```python
from build123d import *
from OCP.BRepFilletAPI import BRepFilletAPI_MakeChamfer

# Parameters (mm, degrees)
F_41_64_0_640630_DIAMETER_HOLE1_D = 16.272002
SKETCH7_W                         = 76.989658396
SKETCH7_H                         = 50.8
FCE_00_BOLT_HEAD_NOTCH_DEPTH      = 50.8
FILLET1_R                         = 3.175
CHAMFER1_SIZE                     = 0.381
CHAMFER1_SIZE2                    = 0.387827593
CUT_EXTRUDE1_DEPTH                = 110.652296603
CUT_EXTRUDE1_DEPTH_BACK           = 110.652296603


with BuildPart() as part:
    # Sketch3 → FBR-00 Basic blank revolve. (revolve)
    with BuildSketch(Plane(origin=(0, 0, 0), x_dir=(0, 0, -1), z_dir=(1, 0, 0)), mode=Mode.PRIVATE) as fbr_00_basic_blank_revolve_sk:
        with BuildLine():
            Line((-101.188905116, 30.1625), (-101.188905116, 0))
            Line((-101.188905116, 0), (-21.038993491, 0))
            Line((-21.038993491, 0), (-6.731, 23.8125))
            Line((-6.731, 23.8125), (9.144, 23.8125))
            Line((9.144, 23.8125), (9.144, 28.448))
            Line((9.144, 28.448), (6.096, 28.448))
            Line((6.096, 28.448), (4.602815367, 26.954815367))
            ThreePointArc((4.602815367, 26.954815367), (4.064, 26.731630735), (3.525184633, 26.954815367))
            Line((3.525184633, 26.954815367), (2.032, 28.448))
            Line((2.032, 28.448), (0, 28.448))
            Line((0, 28.448), (0, 29.21))
            Line((0, 29.21), (-2.286, 29.21))
            Line((-2.286, 29.21), (-3.2385, 30.1625))
            Line((-3.2385, 30.1625), (-101.188905116, 30.1625))
        make_face()
    revolve(fbr_00_basic_blank_revolve_sk.sketch.rotate(Axis((0, 0, -27.766671499), (0, 0, 1)), 90), axis=Axis((0, 0, -27.766671499), (0, 0, 1)))

    # Sketch13 → FCR-00 lacation boss, Cut-Revolve. (revolve, cut)
    with BuildSketch(Plane(origin=(0, 0, 0), x_dir=(0, 0, -1), z_dir=(1, 0, 0))):
        Polygon((-60.009409083, 44.720607894), (-79.306268956, 26.150824711), (-82.534005377, 29.389847768), (-90.632639597, 21.596357919), (-105.074812876, 36.603996473), (-77.621815521, 63.022606131), align=None)
    revolve(axis=Axis((0, 36.603996473, 105.074812876), (0, 0.720551111680328, 0.6934018282758155)), mode=Mode.SUBTRACT)

    # 41/64 (0.640630) Diameter Hole1 (through all)
    with Locations(Plane(origin=(0, 56.495615275, 54.366945365), x_dir=(1, 0, 0), z_dir=(0, 0.720551111680328, 0.6934018282758155))):
        with Locations((0, -50.330495151)):
            Hole(F_41_64_0_640630_DIAMETER_HOLE1_D / 2)

    # FCS-00 End trim, Cut-Sweep: sweep along a path in Sketch6
    with BuildLine(Plane(origin=(0, 53.201255592, 51.196712206), x_dir=(1, 0, 0), z_dir=(0, 0.720551111680328, 0.6934018282758155))) as fcs_00_end_trim_cut_sweep_path:
        Line((-25.4, -39.765602031), (-25.4, -52.465602031))
        ThreePointArc((-25.4, -52.465602031), (-23.103230962, -59.750022773), (-17.04365582, -64.399698315))
        Line((-17.04365582, -64.399698315), (-6.51548373, -68.231639577))
        ThreePointArc((-6.51548373, -68.231639577), (-3.307997785, -69.091082846), (0, -69.380495151))
    # Sketch16 → FCS-00 End trim, Cut-Sweep (sweep, cut)
    with BuildSketch(Plane(origin=(0, 117.771567215, -110.982310617), x_dir=(0, -0.9982398279237649, -0.059306373575968775), z_dir=(-1, 0, 0))):
        with BuildLine():
            Line((152.30720814, 182.06896008), (168.803188567, 201.383271607))
            Line((168.803188567, 201.383271607), (110.860253989, 250.871212889))
            Line((110.860253989, 250.871212889), (88.178280901, 224.314034541))
            Line((88.178280901, 224.314034541), (97.835436664, 216.066044327))
            Line((97.835436664, 216.066044327), (99.302186796, 217.783388083))
            ThreePointArc((99.302186796, 217.783388083), (99.979412877, 218.248832673), (100.798630163, 218.313306472))
            Line((100.798630163, 218.313306472), (112.384771543, 216.165942094))
            Line((112.384771543, 216.165942094), (152.30720814, 182.06896008))
        make_face()
    fcs_00_end_trim_cut_sweep = sweep(path=fcs_00_end_trim_cut_sweep_path.line, mode=Mode.SUBTRACT)

    # FMR-00 Mirror end trim.: FCS-00 End trim, Cut-Sweep across plane
    add(fcs_00_end_trim_cut_sweep.mirror(Plane(origin=(0, 0, 0), x_dir=(0, 0, 1), z_dir=(1, 0, 0))), mode=Mode.SUBTRACT)

    # Sketch7 → FCE-00 Bolt head notch. (cut)
    with BuildSketch(Plane(origin=(0, -18.301998237, 52.237593562), x_dir=(1, 0, 0), z_dir=(0, -0.7205511116803286, -0.6934018282758149))):
        with Locations((0, 6.35)):
            Rectangle(SKETCH7_W, SKETCH7_H)
    extrude(amount=FCE_00_BOLT_HEAD_NOTCH_DEPTH, mode=Mode.SUBTRACT)

    # Fillet1
    fillet1_edges = [part.edges().sort_by_distance(p)[0] for p in [
        (0, -5.092693408, 38.511094884),
    ]]
    fillet(fillet1_edges, radius=FILLET1_R)

    # Chamfer1: one chamfer whose edges measure the first distance from different faces: ONE call of the kernel's chamfer builder (chamfer() names one face for all edges)
    chamfer1_edges_1 = [part.edges().sort_by_distance(p)[0] for p in [
        (28.448, 0, -9.144),
        (23.8125, 0, -9.144),
    ]]
    chamfer1_edges_2 = [part.edges().sort_by_distance(p)[0] for p in [
        (0, 13.80286807, 98.731273817),
    ]]
    chamfer1_side_2 = [part.faces().sort_by_distance(p)[0] for p in [
        (0, 14.023301251, 98.50220985),
    ]]
    chamfer1 = BRepFilletAPI_MakeChamfer(part.part.solid().wrapped)
    for e in chamfer1_edges_1:
        chamfer1.Add(CHAMFER1_SIZE, e.wrapped)
    for e in chamfer1_edges_2:
        chamfer1.Add(CHAMFER1_SIZE, CHAMFER1_SIZE2, e.wrapped, chamfer1_side_2[0].wrapped)  # the first distance lies on this face
    add(Compound.cast(chamfer1.Shape()), mode=Mode.REPLACE)

    # Sketch17 → Cut-Extrude1 (cut, two sides: drawn at the far end of the back side and taken through both)
    with BuildSketch(Plane(origin=(0, 0, 0), x_dir=(0, 0, -1), z_dir=(1, 0, 0)).offset(-CUT_EXTRUDE1_DEPTH_BACK)):
        Polygon((-220.872013196, 249.233244147), (-107.294691274, 15.329981457), (-88.096461038, -24.20721324), (25.480860884, -258.110475929), (-442.325664495, -485.265119773), (-688.678538575, 22.078600303), align=None)
    extrude(amount=CUT_EXTRUDE1_DEPTH + CUT_EXTRUDE1_DEPTH_BACK, mode=Mode.SUBTRACT)


solid = part.part
```
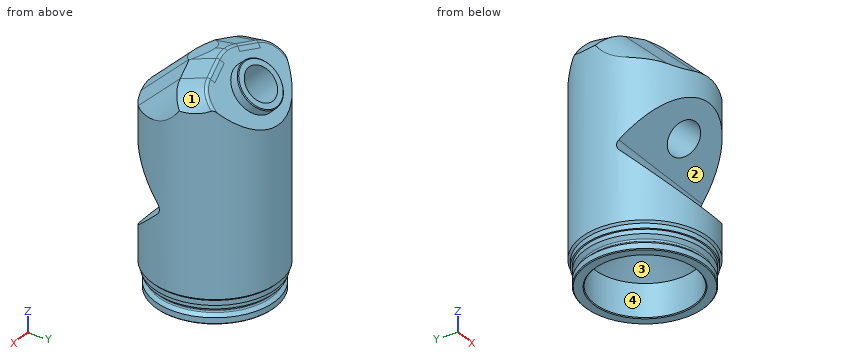
Geometry check sheet. Reference: the model listing, model coordinates, mm. Face numbers are marked on the shaded views. Coordinates: 2 decimals unless noted, no trailing zeros. Loops run counter-clockwise (first coordinate to the right, second up) from the corner with the lowest first, then second, coordinate; pieces in that order, holes last.
Item 1: Go/stop test with flat-tipped pins: pin 1 Ø1.5 at (x, y) = (-10.5, -9.5) entering from +Z; pin 2 Ø6 at (x, y) = (22, 6.5) entering from +Z; pin 3 Ø10 at (x, z) = (18.5, 85.5) entering from +Y. Record where each tip stops, or that it passes through.
Item 2: Thickness scan on line 1 (Z direction, x = 2.5, y = -27); line 2 (Z direction, x = 8, y = -27); line 3 (Y direction, x = 0, z = 3.5). Record the ranges inside material, lowest first.
Item 3: Sectioned sample at A-A, the plane z = 24. Record the boundary of the cut face in (x, y) (1 decimal).
Item 4: Release check for a two-part mould opening along Y. For the marked faces 1, 2, 3 and 4 record: released by +Y, released by -Y, zero draft, split by the parting line, or undercut.
Check result:
1. pin 1: stops at z = 93.73
1. pin 2: stops at z = 96.56
1. pin 3: stops at y = 24.82
2. line 1: z = -9.14 to -4.76, -3.36 to 17.43, 61.28 to 78.95
2. line 2: z = -9.05 to -5.81, -2.32 to 17.43, 61.28 to 77.32
2. line 3: y = -30.16 to -23.81, 23.81 to 30.16
3. outline: (-22.4, -20.2) - (22.4, -20.2) arc R30.2 ccw (long way) to start
4. face 1: split by the parting line
4. face 2: released by -Y
4. face 3: undercut
4. face 4: undercut
